```python
from build123d import *

# Parameters (mm, degrees)
BOSS_EXTRUDE1_DEPTH = 25
SKETCH2_R           = 14
CUT_EXTRUDE1_DEPTH  = 29
CUT_EXTRUDE2_REACH  = 52
SKETCH3_R           = 4


with BuildPart() as part:
    # Sketch1 → Boss-Extrude1 (new body, symmetric)
    with BuildSketch(Plane.XY):
        with BuildLine():
            Line((-25, 0), (25, 0))
            Line((25, 0), (25, -37.113248654))
            Line((25, -37.113248654), (5, -48.660254038))
            ThreePointArc((5, -48.660254038), (0, -50), (-5, -48.660254038))
            Line((-5, -48.660254038), (-25, -37.113248654))
            Line((-25, -37.113248654), (-25, 0))
        make_face()
    extrude(amount=BOSS_EXTRUDE1_DEPTH, both=True)

    # Sketch2 → Cut-Extrude1 (cut)
    with BuildSketch(Plane(origin=(0, 0, 0), x_dir=(1, 0, 0), z_dir=(0, 1, 0))):
        Circle(SKETCH2_R)
    extrude(amount=-CUT_EXTRUDE1_DEPTH, mode=Mode.SUBTRACT)

    # Sketch3 → Cut-Extrude2 (cut, up to next)
    with BuildSketch(Plane.XY.offset(25), mode=Mode.PRIVATE) as cut_extrude2_sk1:
        with Locations((0, -25)):
            Circle(SKETCH3_R)
    cut_extrude2_tool1 = extrude(cut_extrude2_sk1.sketch, amount=-CUT_EXTRUDE2_REACH, mode=Mode.PRIVATE) & part.part
    add(cut_extrude2_tool1.solids().sort_by_distance((0, -25, 25))[0], mode=Mode.SUBTRACT)


solid = part.part
```
Can you work these out from the model? Positions are in its coordinate system, mm. A direction names the side the tool comes from. Coordinates: 2 decimals unless noted, no trailing zeros. Order: outer loops, then holes, each group sorted by start corner. A loop starts at its lowest first (then second) coordinate and runs counter-clockwise, first axis right, second up. Notation, with made-up numbers: (-1, -6.5) -> (11, -6.5) arc R29 cw to (11, 13.5) -> close; hole circle Ø3 at (-29.75, 88). An arc over 180 degrees is marked (long way). Write each question's results on one line, items separated by ' | '.
Item 1: I'm going to push flat-ended pins straight in: pin 1 Ø2 at (y, z) = (-43, -1.5) entering from +X; pin 2 Ø2 at (x, z) = (10.5, 0) entering from -Y; pin 3 Ø10 at (x, z) = (13.5, -11) entering from -Y. Where does each tip first touch, or does it pass through?
Results are:
pin 1: x = 16.54 | pin 2: y = -46.06 | pin 3: y = -46.64
Item 2: Which directions (+Z, -Z, +X, -X, +Y, -Y) give clear straight access to the entire face, cutting with the end or side of a thin tool? Please do faces 1 (the face through (0, -29, 0)), 2 (the face through (0, -19, 25)), 3 (the face through (-0.521, -21.034, 19.289)).
Results are:
face 1: +Y | face 2: +Z, +X, -X, +Y, -Y | face 3: +Z
Item 3: If we mould it in two halves opening along X, with no side actions, what happens to faces 4 (the face through (15.14, -42.806, 0.35)), 5 (the face through (0, -25, -25)), 6 (the face through (7.526, -14.297, -11.805))? For each: +X half, -X half, draft (parallel to the pull), parting line (faces both ways), or undercut.
Results are:
face 4: +X half | face 5: draft | face 6: undercut
Item 4: I want a section at A-A, the plane z = 15. Write out the boundary of the cut face in (x, y).
Results are:
outline: (-25, -37.11) -> (-5, -48.66) arc R10 ccw to (5, -48.66) -> (25, -37.11) -> (25, 0) -> (-25, 0) -> close; hole circle Ø8 at (0, -25)
Item 5: I want a section at C-C, the plane z = 0. Write out the boundary of the cut face in (x, y).
Results are:
outline: (-25, -37.11) -> (-5, -48.66) arc R10 ccw to (5, -48.66) -> (25, -37.11) -> (25, 0) -> (14, 0) -> (14, -29) -> (-14, -29) -> (-14, 0) -> (-25, 0) -> close
Item 6: I want a section at B-B, the plane x = -1. Write out the boundary of the cut face in (y, z).
Results are:
outline: (-49.95, -25) -> (0, -25) -> (0, -13.96) -> (-29, -13.96) -> (-29, 13.96) -> (-28.87, 13.96) -> (-28.87, 25) -> (-49.95, 25) -> close; (-21.13, 13.96) -> (0, 13.96) -> (0, 25) -> (-21.13, 25) -> close
Item 7: If I drill on line 1 along Z through (x, y) = (0, -20); line 2 along X through (y, z) = (-25, 17.5), over which ranges is the centre line in solid material (lowest first)?
Results are:
line 1: -25 to -14, 14 to 25 | line 2: -25 to -4, 4 to 25
Item 8: I want a section at D-D, the plane y = -11.5. Write out the boundary of the cut face in (x, z), then the cut area to 3 significant figures.
Results are:
outline: (-25, -25) -> (25, -25) -> (25, 25) -> (-25, 25) -> close; hole circle Ø28 at (0, 0) | area: 1,880 mm²
